For this review, use the dimensioned drawing (mm, ordinates from the lowest corner) and the shaded views. A direction names the side the tool comes from. Coordinates: 2 decimals unless noted, no trailing zeros. Write each loop counter-clockwise with the first axis right and the second up, starting at its lowest first coordinate (ties: lowest second). Pieces come first, ordered by that corner, then holes.
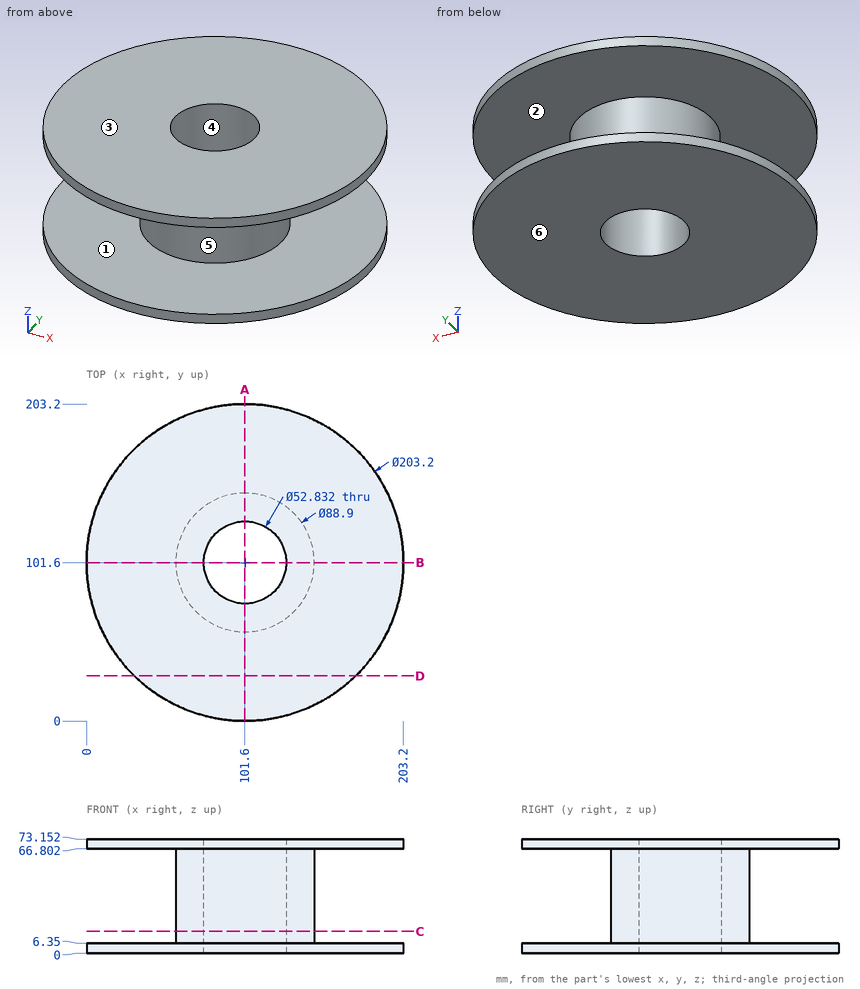
Item 1: Take a section at C-C, the plane z = 14. Write out the cut boundary in (x, y), plus the area to 3 significant figures.
Solved:
outline: circle Ø88.9 at (101.6, 101.6); hole circle Ø52.83 at (101.6, 101.6)
area: 4,010 mm2
Item 2: For pin 1 (1.5 mm diameter, centred on y = 92, z = 36.5, fed in from +X); pin 2 (12 mm diameter, centred on y = 119.5, z = 62, fed in from +X); pin 3 (4 mm diameter, centred on y = 119.5, z = 46.5, fed in from -X), all flat-tipped, find the tip position at first contact; note any pin that passes through.
Solved:
pin 1: stops at x = 145.16
pin 2: stops at x = 202.19
pin 3: stops at x = 60.09
Item 3: Machinability: for the marked faces 5 and 6, which of the approach directions +Z, -Z, +X, -X, +Y, -Y give a long, thin tool a straight path to every point of the face, cutting with its end or side? Answer none if there is none.
Solved:
face 5: none
face 6: -Z, +X, -X, +Y, -Y
Item 4: To check wall thickness, follow line 1 along Z through (x, y) = (141.5, 56.5); line 2 along X through (y, z) = (101, 22); line 3 along Y through (x, z) = (101.5, 42.5). State the ranges of each line that lie inside material, in increasing order.
Solved:
line 1: z = 0 to 6.35, 66.8 to 73.15
line 2: x = 57.15 to 75.19, 128.01 to 146.05
line 3: y = 57.15 to 75.18, 128.02 to 146.05
Item 5: Take a section at D-D, the plane y = 29. Write out the cut boundary in (x, z), plus the area to 3 significant figures.
Solved:
outline: (30.52, 0) - (172.68, 0) - (172.68, 6.35) - (30.52, 6.35) - close; (30.52, 66.8) - (172.68, 66.8) - (172.68, 73.15) - (30.52, 73.15) - close
area: 1,810 mm2
Item 6: Take a section at A-A, the plane x = 101.6. Write out the cut boundary in (y, z).
Solved:
outline: (0, 0) - (75.18, 0) - (75.18, 73.15) - (0, 73.15) - (0, 66.8) - (57.15, 66.8) - (57.15, 6.35) - (0, 6.35) - close; (128.02, 0) - (203.2, 0) - (203.2, 6.35) - (146.05, 6.35) - (146.05, 66.8) - (203.2, 66.8) - (203.2, 73.15) - (128.02, 73.15) - close
Item 7: Mouldability with a two-part tool opening along Z and no side actions: class the marked faces 1, 2, 3 and 4 as pulls with the +Z half, pulls with the -Z half, needs draft (parallel to the pull), parting line crosses it, or undercut.
Solved:
face 1: undercut
face 2: undercut
face 3: pulls with the +Z half
face 4: needs draft
